Could you check a few things on this drawing? It's one solid part, dimensions in mm from its lowest x, y, z. A direction names the side the tool comes from. Coordinates: 2 decimals unless noted, no trailing zeros. Order: outer loops, then holes, each group sorted by start corner. A loop starts at its lowest first (then second) coordinate and runs counter-clockwise, first axis right, second up. Notation, with made-up numbers: (-1.5, 12.25) -> (55.5, 12.25) arc R25 ccw to (55.5, 30.25) -> close; hole circle Ø3 at (68.25, 66.25). An arc over 180 degrees is marked (long way). Answer as CSV lines item,"result".
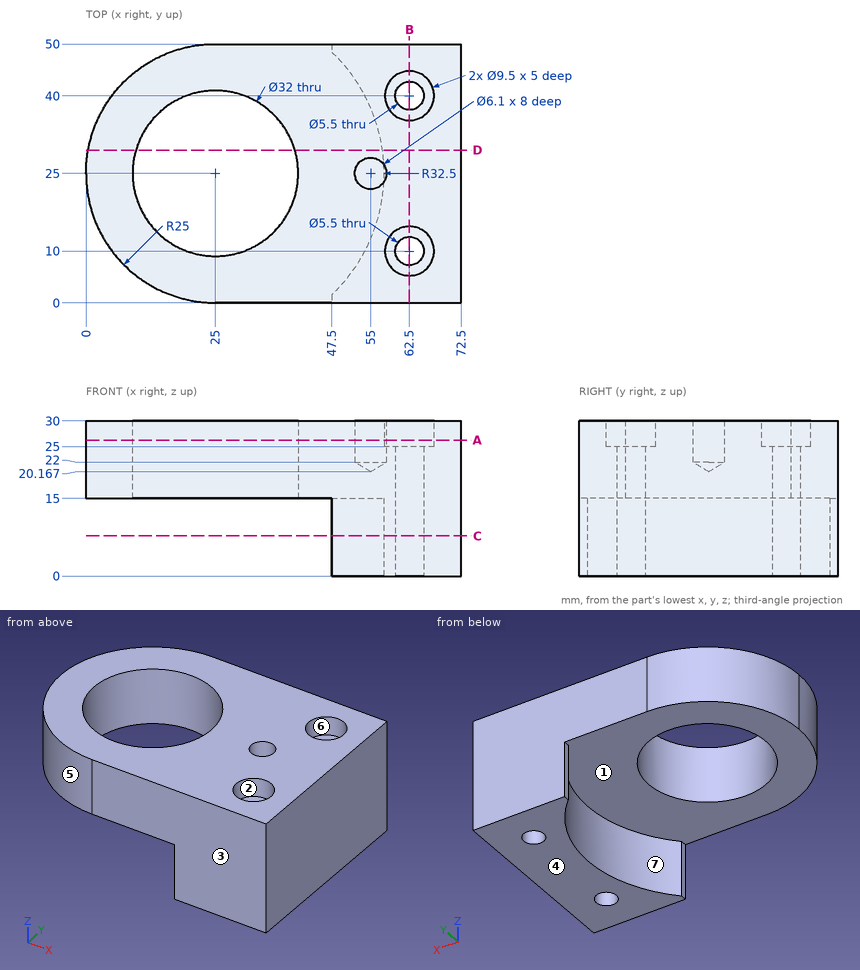
Q1. If I drill on line 1 (Y direction, x = 62.5, z = 6.25); line 2 (Y direction, x = 62.5, z = 28.35); line 3 (Y direction, x = 55, z = 24.75), over which ranges is the centre line in solid material (lowest first)?
Solution:
line 1,"0 to 7.25, 12.75 to 37.25, 42.75 to 50"
line 2,"0 to 5.25, 14.75 to 35.25, 44.75 to 50"
line 3,"0 to 21.95, 28.05 to 50"
Q2. Imagine slicing it at A-A (z = 26.25). Give the number of separate pieces and of enclosed holes in the cut face, and give its area (3 significant figures).
Solution:
separate pieces,"1"
enclosed holes,"4"
area,"2,380 mm2"
Q3. Imagine slicing it at D-D (y = 29.5). List the corners of the cut face in (x, z) for me.
Solution:
outline,"(0.41, 15) -> (9.65, 15) -> (9.65, 30) -> (0.41, 30) -> close; (40.35, 15) -> (57.19, 15) -> (57.19, 0) -> (72.5, 0) -> (72.5, 30) -> (40.35, 30) -> close"
Q4. For P1, Ø8, axis at x = 38, y = 39.5, coming from the -Z side; P2, Ø5, axis at y = 18, z = 15.5, coming from the -X side; P3, Ø7, axis at x = 62.5, y = 10, coming from the +Z side, each with a flat end and sliding along its axis, tell me the tip position at first contact or that it passes through.
Solution:
P1,"z = 15"
P2,"x = 0.41"
P3,"z = 25"
Q5. We'd pull the mould along Y, two halves only. Please class the marked faces 1, 2, 3 and 4: pulls with the +Y half, pulls with the -Y half, needs draft (parallel to the pull), parting line crosses it, or undercut.
Solution:
face 1,"undercut"
face 2,"undercut"
face 3,"pulls with the -Y half"
face 4,"needs draft"
Q6. Which directions (+Z, -Z, +X, -X, +Y, -Y) give clear straight access to the entire face, cutting with the end or side of a thin tool? Please do the marked faces 5, 6 and 7.
Solution:
face 5,"+Z, -Z, -X, -Y"
face 6,"+Z"
face 7,"-Z, -X"
Q7. Imagine slicing it at C-C (z = 7.75). List the corners of the cut face in (x, y) for me.
Solution:
outline,"(47.5, 0) -> (72.5, 0) -> (72.5, 50) -> (47.5, 50) -> (47.5, 48.45) arc R32.5 cw to (47.5, 1.55) -> close; hole circle Ø5.5 at (62.5, 10); hole circle Ø5.5 at (62.5, 40)"
Q8. Imagine slicing it at B-B (x = 62.5). List the corners of the cut face in (y, z) for me.
Solution:
outline,"(0, 0) -> (7.25, 0) -> (7.25, 25) -> (5.25, 25) -> (5.25, 30) -> (0, 30) -> close; (12.75, 0) -> (37.25, 0) -> (37.25, 25) -> (35.25, 25) -> (35.25, 30) -> (14.75, 30) -> (14.75, 25) -> (12.75, 25) -> close; (42.75, 0) -> (50, 0) -> (50, 30) -> (44.75, 30) -> (44.75, 25) -> (42.75, 25) -> close"
